Here's the drawing with two shaded views (mm, measured from the low corner). I have some questions. Give positions to 0.01 mm unless a question says otherwise; leave off trailing zeros. Loops run counter-clockwise (first coordinate to the right, second up) from the corner with the lowest first, then second, coordinate; pieces in that order, holes last.
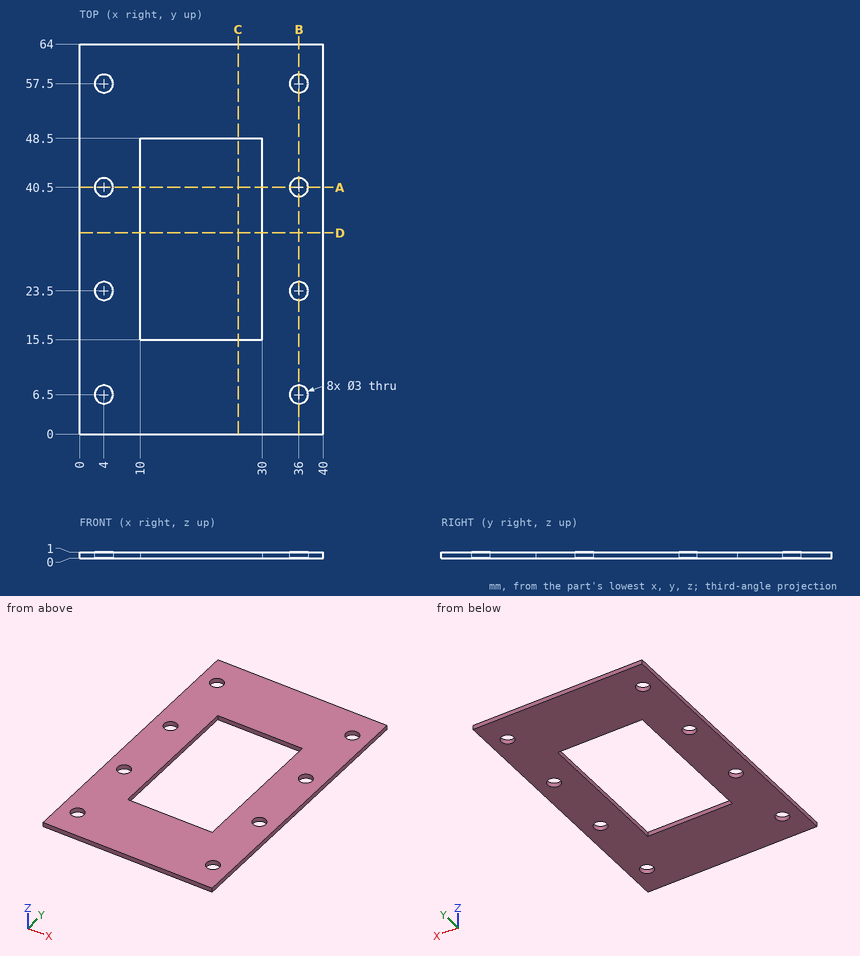
(1) Will this pin go through, and if not, where does the flat tip stop? P1, Ø1.8, axis at x = 4, y = 23.5, coming from the -Z side.
Returned:
P1: passes through
(2) Suppose I cut it at C-C on x = 26. List the corners of the cut face in (y, z) for me.
Returned:
outline: (0, 0) - (15.5, 0) - (15.5, 1) - (0, 1) - close; (48.5, 0) - (64, 0) - (64, 1) - (48.5, 1) - close
(3) Please list where these lines run through material, in increasing order: probe 1 along X at (y, z) = (16.5, 0.4); probe 2 along Y at (x, z) = (4, 0.75); probe 3 along Y at (x, z) = (17, 0.55).
Returned:
probe 1: x = 0 to 10, 30 to 40
probe 2: y = 0 to 5, 8 to 22, 25 to 39, 42 to 56, 59 to 64
probe 3: y = 0 to 15.5, 48.5 to 64
(4) Suppose I cut it at B-B on x = 36. List the corners of the cut face in (y, z) for me, plus the area to 3 significant figures.
Returned:
outline: (0, 0) - (5, 0) - (5, 1) - (0, 1) - close; (8, 0) - (22, 0) - (22, 1) - (8, 1) - close; (25, 0) - (39, 0) - (39, 1) - (25, 1) - close; (42, 0) - (56, 0) - (56, 1) - (42, 1) - close; (59, 0) - (64, 0) - (64, 1) - (59, 1) - close
area: 52.0 mm2
(5) Suppose I cut it at D-D on y = 33. List the corners of the cut face in (x, z) for me, plus the area to 3 significant figures.
Returned:
outline: (0, 0) - (10, 0) - (10, 1) - (0, 1) - close; (30, 0) - (40, 0) - (40, 1) - (30, 1) - close
area: 20.0 mm2
(6) Suppose I cut it at A-A on y = 40.5. List the corners of the cut face in (x, z) for me, plus the area to 3 significant figures.
Returned:
outline: (0, 0) - (2.5, 0) - (2.5, 1) - (0, 1) - close; (5.5, 0) - (10, 0) - (10, 1) - (5.5, 1) - close; (30, 0) - (34.5, 0) - (34.5, 1) - (30, 1) - close; (37.5, 0) - (40, 0) - (40, 1) - (37.5, 1) - close
area: 14.0 mm2
